Part model, mm, in its own coordinate system. Face numbers are marked on the shaded views. A direction names the side the tool comes from. Give positions to 0.01 mm unless a question says otherwise; leave off trailing zeros. Write each loop counter-clockwise with the first axis right and the second up, starting at its lowest first coordinate (ties: lowest second). Pieces come first, ordered by that corner, then holes. Notation, with made-up numbers: M 1.25,51.5 L 15.25,51.5 A14 ccw 15.25,65.5 Z; hole C 31.5,15.5 d6. An arc over 180 degrees is marked long. Use a Markdown table: item, result.
```python
from build123d import *

# Parameters (mm, degrees)
BOSS_EXTRUDE1_DEPTH = 14
HOLE1_D             = 6.5
HOLE2_D             = 6.5
CUT_EXTRUDE1_DEPTH  = 46.814563472
CUT_EXTRUDE2_DEPTH  = 47.465040622
SKETCH8_R           = 3.15
CUT_EXTRUDE3_DEPTH  = 50.746716719
CHAMFER1_SIZE       = 0.5


with BuildPart() as part:
    # Sketch1 → Boss-Extrude1 (new body)
    with BuildSketch(Plane.XY.offset(14)):
        with BuildLine():
            Line((7, 0), (7, 20.267949192))
            Line((7, 20.267949192), (2, 28.92820323))
            Line((2, 28.92820323), (-15.552558883, 39.062177826))
            ThreePointArc((-15.552558883, 39.062177826), (-25.11473671, 36.5), (-22.552558883, 26.937822174))
            Line((-22.552558883, 26.937822174), (-10.464101615, 19.958548116))
            Line((-10.464101615, 19.958548116), (-7, 13.958548116))
            Line((-7, 13.958548116), (-7, 0))
            ThreePointArc((-7, 0), (0, -7), (7, 0))
        make_face()
    extrude(amount=-BOSS_EXTRUDE1_DEPTH)

    # Hole1 (through all)
    with Locations(Plane(origin=(0, 0, 0), x_dir=(-1, 0, 0), z_dir=(0, 0, -1))):
        with Locations((0, 0)):
            Hole(HOLE1_D / 2)

    # Hole2 (through all)
    with Locations(Plane(origin=(0, 0, 0), x_dir=(-1, 0, 0), z_dir=(0, 0, -1))):
        with Locations((19.0525, 32.999898011)):
            Hole(HOLE2_D / 2)

    # Sketch2 → Cut-Extrude1 (cut, through all)
    with BuildSketch(Plane(origin=(6.026279442, 10.437822174, 0), x_dir=(0.8660254037844398, -0.49999999999999806, 0), z_dir=(-0.499999999999998, -0.8660254037844397, 0))):
        with BuildLine():
            Line((-25.999898011, 11.596194078), (-28.29799505, 9.298097039))
            ThreePointArc((-28.29799505, 9.298097039), (-25.999898011, 3.75), (-23.701800972, 9.298097039))
            Line((-23.701800972, 9.298097039), (-25.999898011, 11.596194078))
        make_face()
    extrude(amount=-CUT_EXTRUDE1_DEPTH, mode=Mode.SUBTRACT)

    # Sketch3 → Cut-Extrude2 (cut, through all)
    with BuildSketch(Plane.ZY.offset(7)):
        with BuildLine():
            Line((9.298097039, 4.701902961), (11.596194078, 7))
            Line((11.596194078, 7), (9.298097039, 9.298097039))
            ThreePointArc((9.298097039, 9.298097039), (3.75, 7), (9.298097039, 4.701902961))
        make_face()
    extrude(amount=-CUT_EXTRUDE2_DEPTH, mode=Mode.SUBTRACT)

    # Sketch8 → Cut-Extrude3 (cut, through all)
    with BuildSketch(Plane.XY.offset(14)):
        with Locations((-2.116025404, 20.778312164)):
            Circle(SKETCH8_R)
    extrude(amount=-CUT_EXTRUDE3_DEPTH, mode=Mode.SUBTRACT)

    # Chamfer1
    chamfer1_edges = [part.edges().sort_by_distance(p)[0] for p in [
        (4.5, 24.598076211, 0),
        (-6.776279442, 33.995190528, 0),
        (-25.11473671, 36.5, 0),
        (-16.508330249, 23.448185145, 0),
        (-8.732050808, 16.958548116, 0),
        (-3.25, 0, 0),
        (-7, 6.979274058, 0),
        (-22.3025, 32.999898011, 0),
        (0, -7, 0),
        (-5.266025404, 20.778312164, 0),
        (7, 10.133974596, 0),
    ]]
    chamfer(chamfer1_edges, length=CHAMFER1_SIZE)


solid = part.part
```
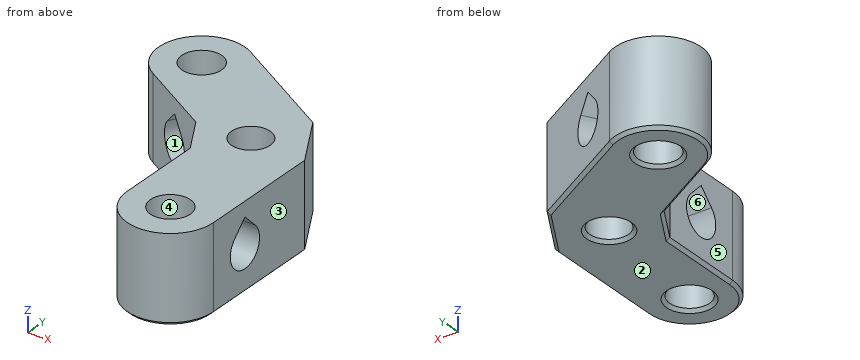
1. Two-plate mould, pull along Z, no slides. Class the marked faces 1, 2 and 3: released by +Z, released by -Z, zero draft, split by the parting line, or undercut.
Findings below:
| item | result |
|---|---|
| face 1 | undercut |
| face 2 | released by -Z |
| face 3 | zero draft |
2. Cut at C-C, the plane z = 11. Give the cut face in (x, y), then the cut area to 3 significant figures.
Findings below:
| item | result |
|---|---|
| outline | M -22.55,26.94 L -17.01,23.74 L -10.01,35.86 L -15.55,39.06 A7 ccw Z; M -15.97,23.14 L -10.46,19.96 L -7,13.96 L -7,7.6 L 7,7.6 L 7,20.27 L 2,28.93 L -8.97,35.26 Z; M -7,0 A7 ccw 7,0 L 7,6.4 L -7,6.4 Z; hole C -19.05,33 d6.5; hole C -2.12,20.78 d6.3; hole C 0,0 d6.5 |
| area | 632 mm2 |
3. Cut at B-B, the plane x = 0. State how many separate pieces and enclosed holes the cut face has, then the cut area to 3 significant figures.
Findings below:
| item | result |
|---|---|
| separate pieces | 3 |
| enclosed holes | 1 |
| area | 327 mm2 |
4. Drill centre lines: L1, parallel to Y at x = -3, z = 12.75; L2, parallel to Y at x = -3, z = 7.25; L3, parallel to X at y = 4.5, z = 11.25. Where is each one in solid material? Low to high.
Findings below:
| item | result |
|---|---|
| L1 | -6.32 to -1.25, 1.25 to 17.75, 23.8 to 31.81 |
| L2 | -6.32 to -1.25, 1.25 to 3.76, 10.24 to 17.75, 23.8 to 31.81 |
| L3 | -7 to 7 |
5. Cut at A-A, the plane z = 5.75. Give the cut face in (x, y), then the cut area to 3 significant figures.
Findings below:
| item | result |
|---|---|
| outline | M -22.55,26.94 L -19.09,24.94 L -12.09,37.06 L -15.55,39.06 A7 ccw Z; M -13.89,21.94 L -10.46,19.96 L -7,13.96 L -7,10 L 7,10 L 7,20.27 L 2,28.93 L -6.89,34.06 Z; M -7,0 A7 ccw 7,0 L 7,4 L -7,4 Z; hole C -19.05,33 d6.5; hole C -2.12,20.78 d6.3; hole C 0,0 d6.5 |
| area | 497 mm2 |
6. Tool access for the marked faces 4, 5 and 6: list every direction of +Z, -Z, +X, -X, +Y, -Y with a clear straight run to the whole face (end or side of a thin tool).
Findings below:
| item | result |
|---|---|
| face 4 | +Z, -Z |
| face 5 | +Z, -Z, -X, -Y |
| face 6 | +X, -X |
7. Drop flat-ended pins along their axis: P1, Ø3, axis at x = -17, z = 10.5, coming from the -Y side; P2, Ø1.5, axis at y = 4.5, z = 4, coming from the -X side; P3, Ø6, axis at y = 7, z = 7, coming from the -X side; P4, Ø6, axis at y = 14.5, z = 7.5, coming from the -X side. Give the stop position or say it passes through.
Findings below:
| item | result |
|---|---|
| P1 | y = 22.87 |
| P2 | x = -7 |
| P3 | through |
| P4 | x = -9.04 |
